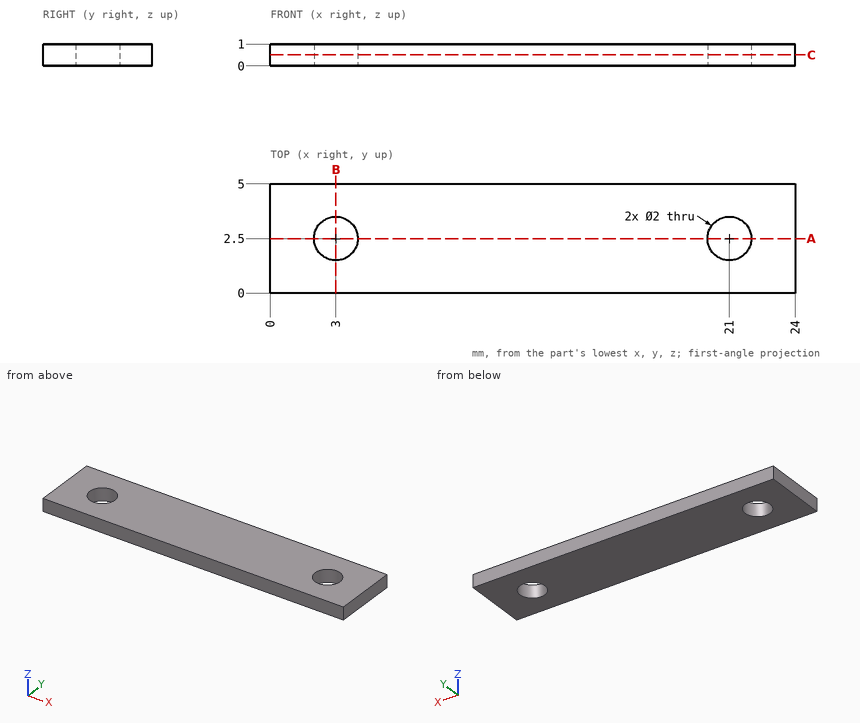
Drawing for the job (mm, zero at the part's lowest x, y, z). Give positions to 0.01 mm unless a question says otherwise; leave off trailing zeros. Loops run counter-clockwise (first coordinate to the right, second up) from the corner with the lowest first, then second, coordinate; pieces in that order, holes last.
(1) Pin check, flat tips, straight feed: pin 1 (2.5 mm diameter, centred on x = 21, y = 2.5, fed in from -Z); pin 2 (1.8 mm diameter, centred on x = 3, y = 2.5, fed in from -Z). Stop position of each tip, or through.
Return value:
pin 1: stops at z = 0
pin 2: passes through
(2) Band-saw the part on A-A (y = 2.5). Write the cut outline in (x, z).
Return value:
outline: (0, 0) - (2, 0) - (2, 1) - (0, 1) - close; (4, 0) - (20, 0) - (20, 1) - (4, 1) - close; (22, 0) - (24, 0) - (24, 1) - (22, 1) - close
(3) Drill centre lines: line 1 along X through (y, z) = (2.5, 0.85); line 2 along Y through (x, z) = (21, 0.4); line 3 along X through (y, z) = (2.05, 0.9). Where is each one in solid material? Low to high.
Return value:
line 1: x = 0 to 2, 4 to 20, 22 to 24
line 2: y = 0 to 1.5, 3.5 to 5
line 3: x = 0 to 2.11, 3.89 to 20.11, 21.89 to 24
(4) Band-saw the part on B-B (x = 3). Write the cut outline in (y, z).
Return value:
outline: (0, 0) - (1.5, 0) - (1.5, 1) - (0, 1) - close; (3.5, 0) - (5, 0) - (5, 1) - (3.5, 1) - close
(5) Band-saw the part on C-C (z = 0.5). Write the cut outline in (x, y).
Return value:
outline: (0, 0) - (24, 0) - (24, 5) - (0, 5) - close; hole circle Ø2 at (3, 2.5); hole circle Ø2 at (21, 2.5)
